Can you work these out from the drawing? Everything is in mm from the part's minimum corner. A direction names the side the tool comes from. Coordinates: 2 decimals unless noted, no trailing zeros. Order: outer loops, then holes, each group sorted by start corner. A loop starts at its lowest first (then second) coordinate and runs counter-clockwise, first axis right, second up. Notation, with made-up numbers: (41.25, 36.25) -> (58.25, 36.25) arc R21 ccw to (58.25, 51.25) -> close; hole circle Ø2 at (-38, -24). An arc over 180 degrees is marked (long way). Put each result on its own line as item: value. Start each with the question number.
Q1. For the marked faces 1, 2, 3 and 4, which set-ups out of +Z, -Z, +X, -X, +Y, -Y let a thin tool reach every point of the face, with its end or its side?
Q2. If we section it at D-D (y = 16): Please give me the cut outline in (x, z) (1 decimal).
Q3. We'd pull the mould along X, two halves only. Please class the marked faces 5, 6, 7 and 8: +X half, -X half, draft (parallel to the pull), parting line (faces both ways), or undercut.
Q4. If we section it at B-B (z = 31.75): Count the separate pieces of the cut face and the enclosed holes in it, and give its area (3 significant figures).
Q5. If we section it at A-A (y = 5.5): Please give me the cut outline in (x, z) (1 decimal), and give its area (3 significant figures).
Q6. Will these pins go through, and if not, where does the flat tip stop? pin 1 (9 mm diameter, centred on y = 13.5, z = 40, fed in from +X) (1 decimal); pin 2 (15 mm diameter, centred on x = 36.51, z = 31.75, fed in from +Y); pin 3 (5 mm diameter, centred on y = 41, z = 26.5, fed in from +X); pin 4 (5 mm diameter, centred on x = 6, z = 28.5, fed in from -Y).
Q7. Please list where these lines run through material, in increasing order: line 1 along Z through (x, y) = (106, 4) (1 decimal); line 2 along X through (y, z) = (5.5, 60.5) (1 decimal); line 3 along X through (y, z) = (8.5, 19.5) (1 decimal).
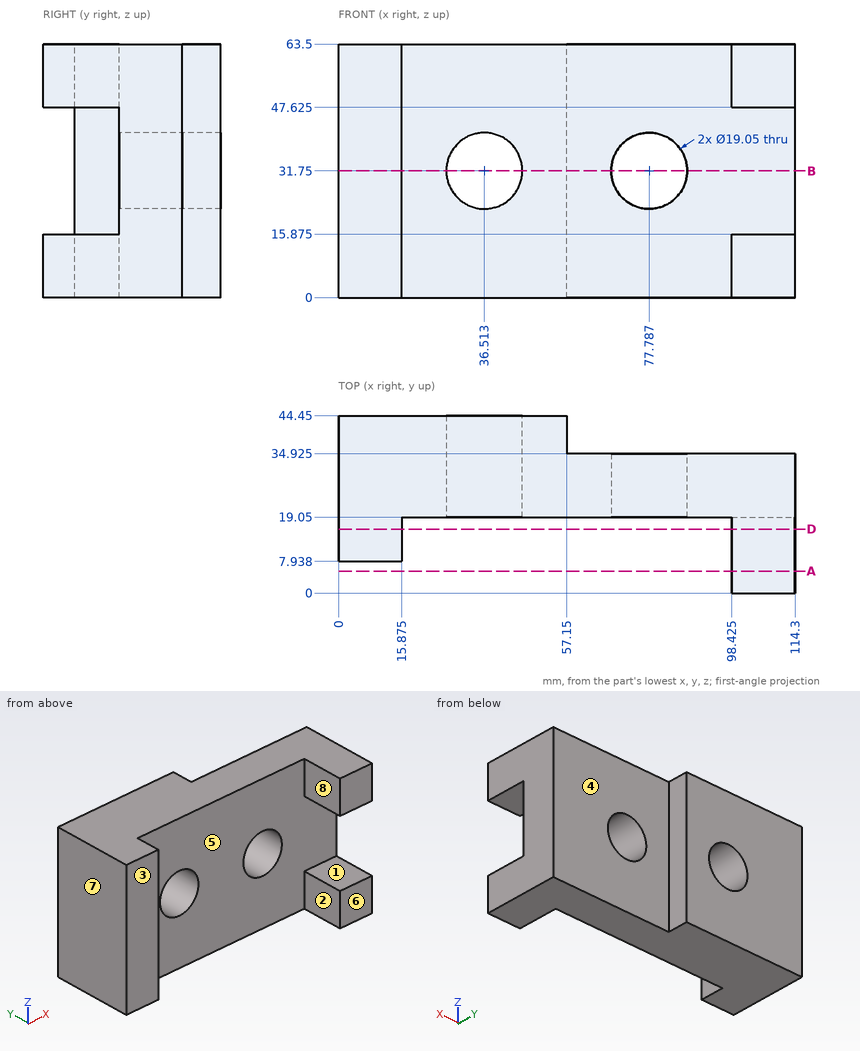
The answers:
1. face 1: +X, -Y
1. face 2: +Z, -Z, -Y
1. face 3: +Z, -Z, -X, -Y
1. face 4: +Z, -Z, +X, +Y
2. outline: (0, 0) -> (15.9, 0) -> (15.9, 63.5) -> (0, 63.5) -> close; (98.4, 0) -> (114.3, 0) -> (114.3, 15.9) -> (98.4, 15.9) -> close; (98.4, 47.6) -> (114.3, 47.6) -> (114.3, 63.5) -> (98.4, 63.5) -> close
3. face 5: undercut
3. face 6: draft
3. face 7: -X half
3. face 8: undercut
4. separate pieces: 3
4. enclosed holes: 0
4. area: 1,750 mm^2
5. outline: (98.4, 0) -> (114.3, 0) -> (114.3, 15.9) -> (98.4, 15.9) -> close; (98.4, 47.6) -> (114.3, 47.6) -> (114.3, 63.5) -> (98.4, 63.5) -> close
5. area: 504 mm^2
6. pin 1: x = 15.9
6. pin 2: through
6. pin 3: x = 57.15
6. pin 4: y = 7.94
7. line 1: 0 to 15.9, 47.6 to 63.5
7. line 2: 98.4 to 114.3
7. line 3: 0 to 15.9
